Verification items for the finished model (mm, model axes). A direction names the side the tool comes from. Give positions to 0.01 mm unless a question says otherwise; leave off trailing zeros. Write each loop counter-clockwise with the first axis right and the second up, starting at its lowest first coordinate (ties: lowest second). Pieces come first, ordered by that corner, then holes.
from build123d import *

# Parameters (mm, degrees)
SKETCH1_W           = 3.81
SKETCH1_H           = 5.08
BOSS_EXTRUDE1_DEPTH = 5.08
CUT_EXTRUDE1_DEPTH  = 5.08


with BuildPart() as part:
    # Sketch1 → Boss-Extrude1 (new body)
    with BuildSketch(Plane(origin=(0, 0, 0), x_dir=(1, 0, 0), z_dir=(0, 1, 0))):
        Polygon((-2.995905159, -37.721169498), (26.791971131, -16.079010555), (15.414014841, 18.938738206), (-21.405825159, 18.938738206), (-32.783781449, -16.079010555), align=None)
        Polygon((15.238089821, -3.146472779), (16.415444569, -6.769998106), (11.584077466, -8.339804437), (10.406722718, -4.71627911), align=None, mode=Mode.SUBTRACT)
        with Locations((1.449094841, 9.40671805)):
            Rectangle(SKETCH1_W, SKETCH1_H, mode=Mode.SUBTRACT)
        with Locations((-7.440905159, 9.40671805)):
            Rectangle(SKETCH1_W, SKETCH1_H, mode=Mode.SUBTRACT)
        Polygon((13.668283489, 1.684894324), (12.490928741, 5.308419651), (7.659561638, 3.73861332), (8.836916386, 0.115087993), align=None, mode=Mode.SUBTRACT)
        Polygon((5.733323489, -22.736401436), (2.650968741, -24.975863247), (-0.334980341, -20.866056916), (2.747374408, -18.626595105), align=None, mode=Mode.SUBTRACT)
        Polygon((9.843129821, -19.750452355), (12.925484569, -17.510990543), (9.939535488, -13.401184212), (6.857180739, -15.640646023), align=None, mode=Mode.SUBTRACT)
        Polygon((-15.834940138, -19.750452355), (-18.917294887, -17.510990543), (-15.931345805, -13.401184212), (-12.848991056, -15.640646023), align=None, mode=Mode.SUBTRACT)
        Polygon((-11.725133807, -22.736401436), (-8.642779058, -24.975863247), (-5.656829976, -20.866056916), (-8.739184725, -18.626595105), align=None, mode=Mode.SUBTRACT)
        Polygon((-19.660093807, 1.684894324), (-18.482739058, 5.308419651), (-13.651371955, 3.73861332), (-14.828726704, 0.115087993), align=None, mode=Mode.SUBTRACT)
        Polygon((-21.229900138, -3.146472779), (-22.407254887, -6.769998106), (-17.575887784, -8.339804437), (-16.398533035, -4.71627911), align=None, mode=Mode.SUBTRACT)
    extrude(amount=BOSS_EXTRUDE1_DEPTH)

    # Sketch2 → Cut-Extrude1 (cut)
    with BuildSketch(Plane(origin=(0, 5.08, 0), x_dir=(1, 0, 0), z_dir=(0, 1, 0))):
        Polygon((-2.995905159, 1.219657161), (-0.455905159, 1.219657161), (-0.455905159, -3.860342839), (4.624094841, -3.860342839), (4.624094841, -6.400342839), (4.624094841, -8.940342839), (-0.455905159, -8.940342839), (-0.455905159, -14.020342839), (-2.995905159, -14.020342839), (-5.535905159, -14.020342839), (-5.535905159, -8.940342839), (-10.615905159, -8.940342839), (-10.615905159, -6.400342839), (-10.615905159, -3.860342839), (-5.535905159, -3.860342839), (-5.535905159, 1.219657161), align=None)
    extrude(amount=-CUT_EXTRUDE1_DEPTH, mode=Mode.SUBTRACT)


solid = part.part
Item 1: Sectioned sample at C-C on y = 2.55. State how many separate pieces and enclosed holes the cut face has, then the cut area to 3 significant figures.
Answer key:
separate pieces: 1
enclosed holes: 11
area: 2,010 mm2
Item 2: Sectioned sample at B-B on x = -7. Record the cut outline in (y, z).
Answer key:
outline: (0, -18.94) - (5.08, -18.94) - (5.08, -11.95) - (0, -11.95) - close; (0, -6.87) - (5.08, -6.87) - (5.08, 3.86) - (0, 3.86) - close; (0, 8.94) - (5.08, 8.94) - (5.08, 19.89) - (0, 19.89) - close; (0, 22.71) - (5.08, 22.71) - (5.08, 34.81) - (0, 34.81) - close
Item 3: Depth check by flat-ended pin: pin 1 (2 mm diameter, centred on y = 1, z = 19, fed in from -X); pin 2 (2.5 mm diameter, centred on y = 1.5, z = 10.5, fed in from -X); pin 3 (10 mm diameter, centred on x = 14, z = -10.5, fed in from -Y); pin 4 (1.1 mm diameter, centred on x = -8, y = 3.5, fed in from +Z). Enter the tip coordinate at first touch or a pass-through.
Answer key:
pin 1: stops at x = -30.14
pin 2: stops at x = -31.38
pin 3: stops at y = 0
pin 4: stops at z = 34.49
Item 4: Sectioned sample at D-D on z = 12.5. Record the cut outline in (x, y), then the cut area to 3 significant figures.
Answer key:
outline: (-31.62, 0) - (-5.54, 0) - (-5.54, 5.08) - (-31.62, 5.08) - close; (-0.46, 0) - (25.63, 0) - (25.63, 5.08) - (-0.46, 5.08) - close
area: 265 mm2
Item 5: Sectioned sample at A-A on z = 1. Record the cut outline in (x, y), then the cut area to 3 significant figures.
Answer key:
outline: (-27.88, 0) - (-5.54, 0) - (-5.54, 5.08) - (-27.88, 5.08) - close; (-0.46, 0) - (21.89, 0) - (21.89, 5.08) - (-0.46, 5.08) - close
area: 227 mm2
Item 6: Set-up check for faces 4 (the face through (11.69, 2.5, 27.05)), 5 (the face through (-7.17, 2.5, 22.95)): record each of +Z, -Z, +X, -X, +Y, -Y from which the full face is reachable in a straight line by a thin tool's end or side.
Answer key:
face 4: +Z, +X, +Y, -Y
face 5: +Y, -Y
Item 7: Release check for a two-part mould opening along Z. For faces 1 (the face through (-18.098, 2.504, 26.749)), 2 (the face through (8.24, 2.5, -1.95)), 3 (the face through (21.183, 2.504, -1.185)) record: released by +Z, released by -Z, zero draft, split by the parting line, or undercut.
Answer key:
face 1: released by +Z
face 2: undercut
face 3: released by -Z
Item 8: Scan lines: line 1 along X through (y, z) = (2.65, 5); line 2 along Z through (x, y) = (-16, 4.7); line 3 along X through (y, z) = (2.9, 23). Record each from-to range of solid material in increasing order.
Answer key:
line 1: x = -29.18 to -21.83, -16.49 to -10.62, 4.62 to 10.5, 15.84 to 23.19
line 2: z = -18.94 to -4.5, -0.5 to 13.5, 19.63 to 28.27
line 3: x = -23.26 to -11.36, -7.21 to 1.22, 5.37 to 17.27
